Can you work these out from the model? Positions are in its coordinate system, mm. A direction names the side the tool comes from. Give positions to 0.01 mm unless a question says otherwise; leave off trailing zeros. Write each loop counter-clockwise with the first axis right and the second up, starting at its lowest first coordinate (ties: lowest second). Pieces come first, ordered by that corner, then holes. Notation, with made-up numbers: M -40,-20.75 L -11,-20.75 A31 ccw -11,3.25 Z; hole C 57,-1 d9. An arc over 180 degrees is marked long. Write each question's results on one line, items separated by ' | '.
from build123d import *

# Parameters (mm, degrees)
SZKIC1_R                    = 10
DODANIE_WYCI_GNI_CIE1_DEPTH = 105
SZKIC2_R                    = 5
DODANIE_WYCI_GNI_CIE2_DEPTH = 50
WYTNIJ_WYCI_GNI_CIE1_DEPTH  = 2
SFAZOWANIE1_SIZE            = 1
SFAZOWANIE2_SIZE            = 2
SFAZOWANIE3_SIZE            = 1
SZKIC5_W                    = 1
SZKIC5_H                    = 1.2


with BuildPart() as part:
    # Szkic1 → Dodanie-wyciągnięcie1 (new body)
    with BuildSketch(Plane.XY):
        Circle(SZKIC1_R)
    extrude(amount=DODANIE_WYCI_GNI_CIE1_DEPTH)

    # Szkic2 → Dodanie-wyciągnięcie2 (add)
    with BuildSketch(Plane.XY.offset(105)):
        Circle(SZKIC2_R)
    extrude(amount=DODANIE_WYCI_GNI_CIE2_DEPTH)

    # Szkic3 → Wytnij-wyciągnięcie1 (cut)
    with BuildSketch(Plane(origin=(0, 5, 0), x_dir=(1, 0, 0), z_dir=(0, 1, 0))):
        with BuildLine():
            Line((-1.5, -151.5), (-1.5, -146.5))
            ThreePointArc((-1.5, -146.5), (0, -145), (1.5, -146.5))
            Line((1.5, -146.5), (1.5, -151.5))
            ThreePointArc((1.5, -151.5), (0, -153), (-1.5, -151.5))
        make_face()
    extrude(amount=-WYTNIJ_WYCI_GNI_CIE1_DEPTH, mode=Mode.SUBTRACT)

    # Sfazowanie1
    sfazowanie1_edges = [part.edges().sort_by_distance(p)[0] for p in [
        (-5, 0, 105),
    ]]
    chamfer(sfazowanie1_edges, length=SFAZOWANIE1_SIZE)

    # Sfazowanie2
    sfazowanie2_edges = [part.edges().sort_by_distance(p)[0] for p in [
        (-10, 0, 105),
    ]]
    chamfer(sfazowanie2_edges, length=SFAZOWANIE2_SIZE)

    # Sfazowanie3
    sfazowanie3_edges = [part.edges().sort_by_distance(p)[0] for p in [
        (-5, 0, 155),
    ]]
    chamfer(sfazowanie3_edges, length=SFAZOWANIE3_SIZE)

    # Szkic5 → Wycięcie-obrót1 (revolve, cut)
    with BuildSketch(Plane(origin=(0, 0, 0), x_dir=(1, 0, 0), z_dir=(0, 1, 0)), mode=Mode.PRIVATE) as wyci_cie_obr_t1_sk:
        with Locations((-9.5, -74.4)):
            Rectangle(SZKIC5_W, SZKIC5_H)
    revolve(wyci_cie_obr_t1_sk.sketch.rotate(Axis((0, 0, 106), (0, 0, -1)), 180), axis=Axis((0, 0, 106), (0, 0, -1)), mode=Mode.SUBTRACT)


solid = part.part
Item 1: I want a section at B-B, the plane y = 0. Please give me the cut outline in (x, z), and give its area (3 significant figures).
Geometry says:
outline: M -10,0 L 10,0 L 10,73.8 L 9,73.8 L 9,75 L 10,75 L 10,103 L 8,105 L 6,105 L 5,106 L 5,154 L 4,155 L -4,155 L -5,154 L -5,106 L -6,105 L -8,105 L -10,103 L -10,75 L -9,75 L -9,73.8 L -10,73.8 Z | area: 2,590 mm2
Item 2: For faces 5 (the face through (-1.08, -4.88, 129.66)), 6 (the face through (-2.17, -9.76, 36.38)), 7 (the face through (-9, -2, 73.8)), which set-ups out of +Z, -Z, +X, -X, +Y, -Y let a thin tool reach every point of the face, with its end or its side?
Geometry says:
face 5: +Z | face 6: +Z, -Z | face 7: none
Item 3: I want a section at C-C, the plane z = 63.5. Please give me the cut outline in (x, y).
Geometry says:
outline: C 0,0 d20
Item 4: I'm going to push flat-ended pins straight in: pin 1 (2 mm diameter, centred on y = -5, z = 112.5, fed in from +X); pin 2 (10 mm diameter, centred on y = 7, z = 70, fed in from -X); pin 3 (1.4 mm diameter, centred on y = 4, z = 150, fed in from -X). Where does each tip first touch, or does it pass through?
Geometry says:
pin 1: stops at x = 3 | pin 2: stops at x = -9.8 | pin 3: stops at x = -3.76
Item 5: I want a section at D-D, the plane z = 127. Please give me the cut outline in (x, y), and give its area (3 significant figures).
Geometry says:
outline: C 0,0 d10 | area: 78.5 mm2
Item 6: Thinking about a two-plate mould opening in Z: for faces 1 (the face through (-2, 6, 105)), 2 (the face through (0, 3, 149)), 3 (the face through (-9, -2, 75)), 4 (the face through (-2.17, -9.76, 88.8)), which applies, +Z half, -Z half, draft (parallel to the pull), parting line (faces both ways), or undercut?
Geometry says:
face 1: +Z half | face 2: undercut | face 3: undercut | face 4: draft
Item 7: I want a section at A-A, the plane x = 0. Please give me the cut outline in (y, z).
Geometry says:
outline: M -10,0 L 10,0 L 10,73.8 L 9,73.8 L 9,75 L 10,75 L 10,103 L 8,105 L 6,105 L 5,106 L 5,145 L 3,145 L 3,153 L 5,153 L 5,154 L 4,155 L -4,155 L -5,154 L -5,106 L -6,105 L -8,105 L -10,103 L -10,75 L -9,75 L -9,73.8 L -10,73.8 Z
Item 8: If I drill on line 1 (Z direction, x = 5.5, y = 3.75); line 2 (Z direction, x = -1, y = 4.75); line 3 (X direction, y = -0.25, z = 50.5), over which ranges is the centre line in solid material (lowest first)? Write a range as from..to.
Geometry says:
line 1: z = 0..105 | line 2: z = 0..145.38, 152.62..154.15 | line 3: x = -10..10
